The figure shows three views and two pictorial views of one solid part (mm, origin at its lowest corner). Answer the questions. A direction names the side the tool comes from. Coordinates: 2 decimals unless noted, no trailing zeros. Order: outer loops, then holes, each group sorted by start corner. A loop starts at its lowest first (then second) coordinate and runs counter-clockwise, first axis right, second up. Notation, with made-up numbers: (33.5, 23) -> (50.5, 23) arc R17 cw to (50.5, 30) -> close; hole circle Ø6 at (44, 80.25). An arc over 180 degrees is marked (long way). Return JSON: item names as keys, results as strings.
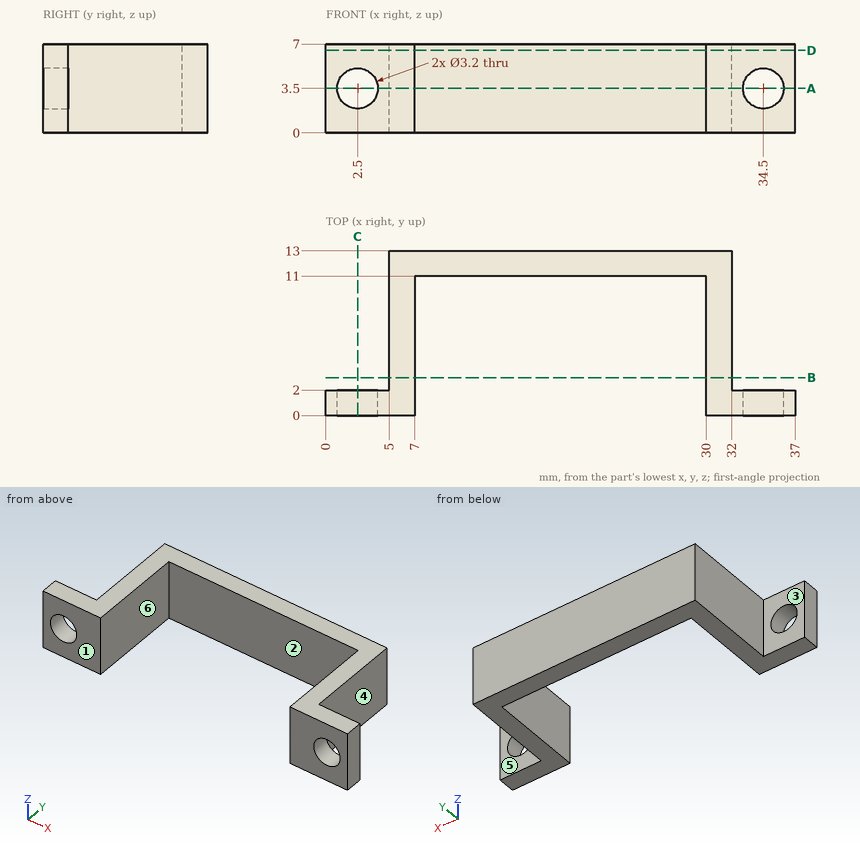
1. The part is cut by section A-A on z = 3.5. Give the vertices of the cut face in (x, y).
Answer block:
{"outline": "(0, 0) -> (0.9, 0) -> (0.9, 2) -> (0, 2) -> close; (4.1, 0) -> (7, 0) -> (7, 11) -> (30, 11) -> (30, 0) -> (32.9, 0) -> (32.9, 2) -> (32, 2) -> (32, 13) -> (5, 13) -> (5, 2) -> (4.1, 2) -> close; (36.1, 0) -> (37, 0) -> (37, 2) -> (36.1, 2) -> close"}
2. For the marked faces 1, 2 and 3, determine the directions among +Z, -Z, +X, -X, +Y, -Y from which every point of the face is accessible in a straight line to the end or side of a thin tool.
Answer block:
{"face 1": "+Z, -Z, +X, -X, -Y", "face 2": "+Z, -Z, -Y", "face 3": "+Z, -Z, -X, +Y"}
3. Determine the mould class of the marked faces 4, 5 and 6 for opening direction X: pulls with the +X half, pulls with the -X half, needs draft (parallel to the pull), parting line crosses it, or undercut.
Answer block:
{"face 4": "pulls with the +X half", "face 5": "needs draft", "face 6": "undercut"}
4. Each of these flat-tipped pins is pushed along its axis until it touches: pin 1 Ø2 at (x, z) = (19, 2.5) entering from -Y; pin 2 Ø2.5 at (x, z) = (34.5, 4.5) entering from +Y; pin 3 Ø2 at (y, z) = (4, 4) entering from +X. Where does it stop, or does it pass through?
Answer block:
{"pin 1": "stops at y = 11", "pin 2": "stops at y = 2", "pin 3": "stops at x = 32"}
5. The part is cut by section B-B on y = 3. Give the vertices of the cut face in (x, z).
Answer block:
{"outline": "(5, 0) -> (7, 0) -> (7, 7) -> (5, 7) -> close; (30, 0) -> (32, 0) -> (32, 7) -> (30, 7) -> close"}
6. The part is cut by section D-D on z = 6.5. Give the vertices of the cut face in (x, y).
Answer block:
{"outline": "(0, 0) -> (7, 0) -> (7, 11) -> (30, 11) -> (30, 0) -> (37, 0) -> (37, 2) -> (32, 2) -> (32, 13) -> (5, 13) -> (5, 2) -> (0, 2) -> close"}
7. The part is cut by section C-C on x = 2.5. Give the vertices of the cut face in (y, z).
Answer block:
{"outline": "(0, 0) -> (2, 0) -> (2, 1.9) -> (0, 1.9) -> close; (0, 5.1) -> (2, 5.1) -> (2, 7) -> (0, 7) -> close"}
8. Consider line 1 (X direction, y = 0.65, z = 3.5); line 2 (X direction, y = 4, z = 6.25); line 3 (Y direction, x = 4.5, z = 1.25). Determine where each line is inside the solid, lowest interval first. Write a range as from..to.
Answer block:
{"line 1": "x = 0..0.9, 4.1..7, 30..32.9, 36.1..37", "line 2": "x = 5..7, 30..32", "line 3": "y = 0..2"}
